from build123d import *

# Parameters (mm, degrees)
F0_R     = 23.4400047289
F1_DEPTH = 28
F3_R     = 17.0810137282
F4_DEPTH = 9
F5_T     = -8
F6_D     = 10


with BuildPart() as f1:
    # F0 (on Front) → F1 (new body)
    with BuildSketch(Plane.XZ):
        with Locations((0, 23.6968044192)):
            Circle(F0_R)
    extrude(amount=F1_DEPTH)


with BuildPart() as f1_1:
    # F2: moved
    add(f1.part.moved(Location((0, 25.654, 0))))

    # F3 (on face) → F4 (join)
    with BuildSketch(Plane.XZ.offset(2.346)):
        with Locations((0, 23.6968044192)):
            Circle(F3_R)
    extrude(amount=F4_DEPTH)

    # F5
    f5_openings = [f1_1.faces().sort_by_distance(p)[0] for p in [
        (0, -11.346, 23.696804),
    ]]
    offset(amount=F5_T, openings=f5_openings, kind=Kind.INTERSECTION)

    # F6 (through all)
    with Locations(Plane.XZ):
        with Locations((0, 23.6968044192)):
            Hole(F6_D / 2)


solid = f1_1.part
Can you work these out from the model? Positions are in its coordinate system, mm. A direction names the side the tool comes from. Give positions to 0.01 mm unless a question says otherwise; leave off trailing zeros. Loops run counter-clockwise (first coordinate to the right, second up) from the corner with the lowest first, then second, coordinate; pieces in that order, holes last. Notation, with made-up numbers: M 37.25,-34 L 91.25,-34 A10 cw 91.25,-29 Z; hole C 71.5,11.25 d4. An arc over 180 degrees is marked long. One line per item, written item: value.
1) Please list where these lines run through material, in increasing order: line 1 (Y direction, x = -0.5, z = 37.5); line 2 (Z direction, x = 0, y = 15); line 3 (Z direction, x = 0, y = 1).
Geometry check:
line 1: y = -11.35 to 5.65, 17.65 to 25.65
line 2: z = 0.26 to 8.26, 39.14 to 47.14
line 3: z = 0.26 to 14.62, 32.78 to 47.14
2) Imagine slicing it at D-D on z = 12.5. Write out the boundary of the cut face in (x, y).
Geometry check:
outline: M -20.59,-2.35 L -12.9,-2.35 L -12.9,-11.35 L 12.9,-11.35 L 12.9,-2.35 L 20.59,-2.35 L 20.59,25.65 L -20.59,25.65 Z; hole M -10.63,5.65 L 10.63,5.65 L 10.63,17.65 L -10.63,17.65 Z
3) I'm going to push flat-ended pins straight in: pin 1 (4 mm diameter, centred on x = 14, y = 13.5, fed in from +Z); pin 2 (16 mm diameter, centred on x = 0, z = 23.7, fed in from -Y); pin 3 (1.5 mm diameter, centred on y = -0.5, z = 29, fed in from +X). Where does each tip first touch, or does it pass through?
Geometry check:
pin 1: stops at z = 43.83
pin 2: stops at y = 17.65
pin 3: stops at x = 22.99
4) On a 3-axis mill with a long thin cutter (end or side, diameter ignored), from which of +Z, -Z, +X, -X, +Y, -Y can I reach the whole of each face in a straight line? I mean faces 1 (the face through (7, 5.654, 17)), 2 (the face through (0.651, 21.71, 28.654)), 3 (the face through (2, -2.346, 6)). Say none if no direction works.
Geometry check:
face 1: none
face 2: +Y, -Y
face 3: -Y
5) Imagine slicing it at C-C on z = 17.5. Write out the boundary of the cut face in (x, y).
Geometry check:
outline: M -22.61,-2.35 L -15.92,-2.35 L -15.92,-11.35 L -6.64,-11.35 L -6.64,5.65 L -14.14,5.65 L -14.14,17.65 L 14.14,17.65 L 14.14,5.65 L 6.64,5.65 L 6.64,-11.35 L 15.92,-11.35 L 15.92,-2.35 L 22.61,-2.35 L 22.61,25.65 L -22.61,25.65 Z
6) Imagine slicing it at A-A on x = 0. Write out the boundary of the cut face in (y, z), and give its area (3 significant figures).
Geometry check:
outline: M -11.35,6.62 L -2.35,6.62 L -2.35,0.26 L 25.65,0.26 L 25.65,18.7 L 17.65,18.7 L 17.65,8.26 L 5.65,8.26 L 5.65,14.62 L -11.35,14.62 Z; M -11.35,32.78 L 5.65,32.78 L 5.65,39.14 L 17.65,39.14 L 17.65,28.7 L 25.65,28.7 L 25.65,47.14 L -2.35,47.14 L -2.35,40.78 L -11.35,40.78 Z
area: 861 mm²
7) Imagine slicing it at B-B on x = -14. Write out the boundary of the cut face in (y, z), and give its area (3 significant figures).
Geometry check:
outline: M -11.35,13.91 L -2.35,13.91 L -2.35,4.9 L 25.65,4.9 L 25.65,42.5 L -2.35,42.5 L -2.35,33.48 L -11.35,33.48 Z; hole M 5.65,17.19 L 17.65,17.19 L 17.65,30.21 L 5.65,30.21 Z
area: 1,070 mm²
8) Thinking about a two-plate mould opening in Z: for faces 4 (the face through (-1.97, -2.73, 14.83)), 5 (the face through (-18.6, 11.85, 9.43)), 6 (the face through (0, 25.654, 29)), which applies, +Z half, -Z half, draft (parallel to the pull), parting line (faces both ways), or undercut?
Geometry check:
face 4: undercut
face 5: parting line
face 6: draft
